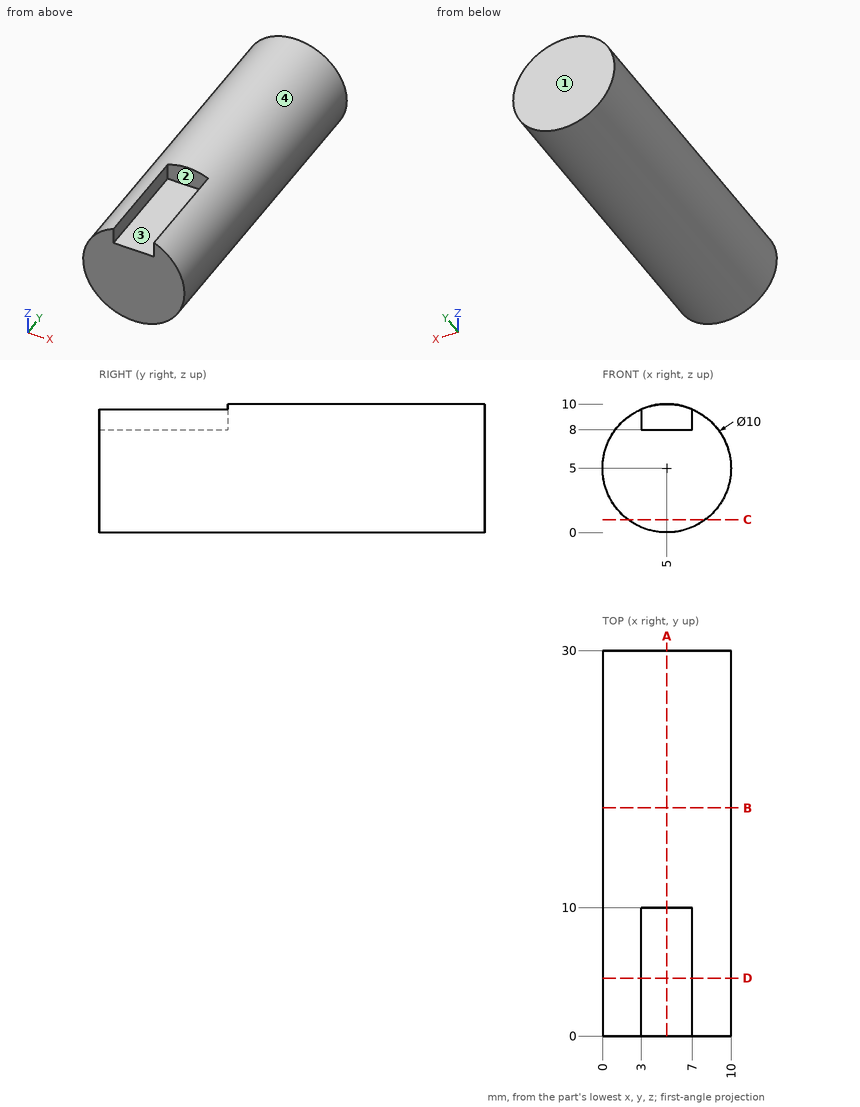
Study the drawing (mm; zero at the part's minimum x, y, z) and answer. Coordinates: 2 decimals unless noted, no trailing zeros. Loops run counter-clockwise (first coordinate to the right, second up) from the corner with the lowest first, then second, coordinate; pieces in that order, holes last. Notation, with made-up numbers: M 86.25,55 L 123.25,55 A19 cw 123.25,59 Z; hole C 42.5,-10 d10. An arc over 180 degrees is marked long. Answer in a Markdown table with one row per item. Add a question column.
1. The mould has two halves that part along X. Classify the marked faces 1, 2, 3 and 4: pulls with the +X half, pulls with the -X half, needs draft (parallel to the pull), parting line crosses it, or undercut.
2. Find section A-A, the plane x = 5. Write down the section's boundary in (y, z), then the cut area to 3 significant figures.
3. Flat-ended cylindrical pins translate along their axes: P1, Ø0.5, axis at y = 4, z = 8.5, coming from the -X side; P2, Ø5, axis at y = 17.5, z = 4, coming from the +X side; P3, Ø1, axis at x = 6, y = 5, coming from the -Z side; P4, Ø4.5, axis at x = 4.5, y = 5, coming from the +Z side. Find the tip coordinate at first contact, or state that the pin passes through.
4. Find section B-B, the plane y = 17.75. Write down the section's boundary in (x, z), then the cut area to 3 significant figures.
5. Find section C-C, the plane z = 1. Write down the section's boundary in (x, y), then the cut area to 3 significant figures.
6. Find section D-D, the plane y = 4.5. Write down the section's boundary in (x, z).
Reported:
| question | item | result |
|---|---|---|
| 1 | face 1 | needs draft |
| 1 | face 2 | undercut |
| 1 | face 3 | undercut |
| 1 | face 4 | parting line crosses it |
| 2 | outline | M 0,0 L 30,0 L 30,10 L 10,10 L 10,8 L 0,8 Z |
| 2 | area | 280 mm^2 |
| 3 | P1 | stops at x = 1.2 |
| 3 | P2 | stops at x = 10 |
| 3 | P3 | stops at z = 0.03 |
| 3 | P4 | stops at z = 9.58 |
| 4 | outline | C 5,5 d10 |
| 4 | area | 78.5 mm^2 |
| 5 | outline | M 2,0 L 8,0 L 8,30 L 2,30 Z |
| 5 | area | 180 mm^2 |
| 6 | outline | M 3,8 L 3,9.58 A5 ccw long 7,9.58 L 7,8 Z |
